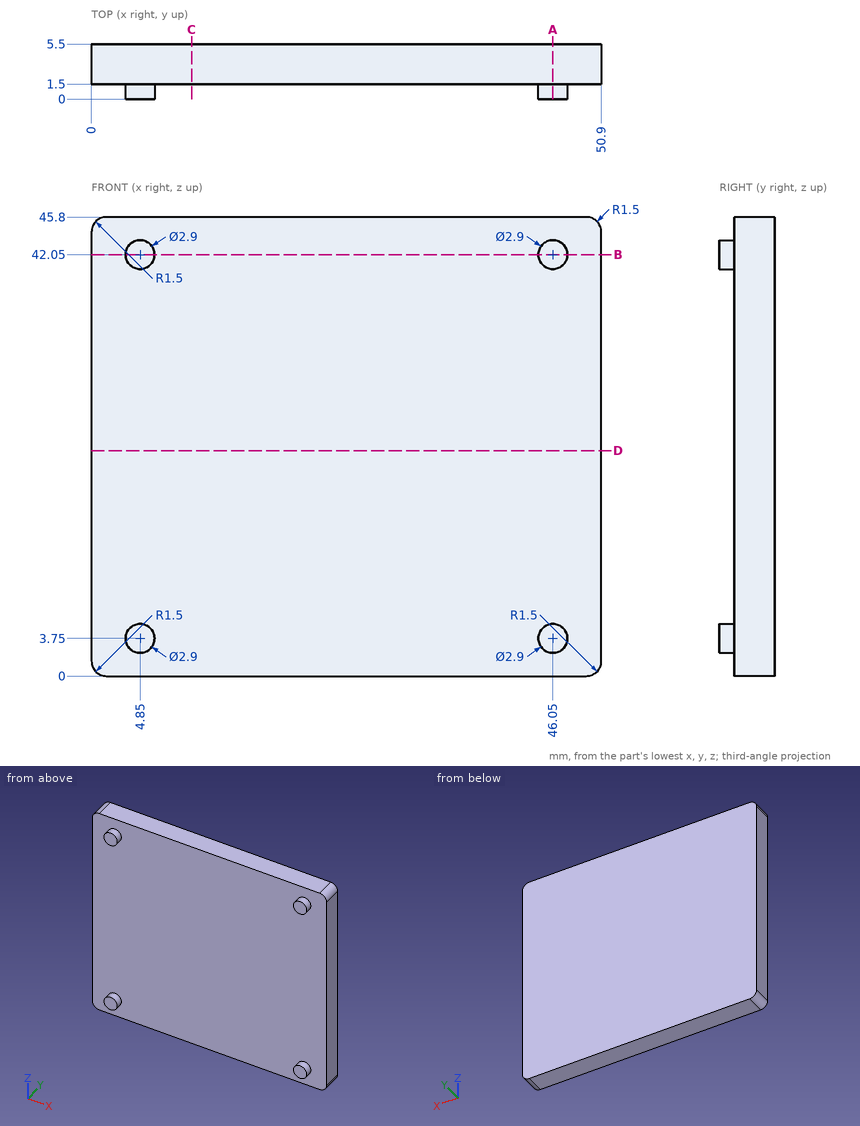
Job drawing, mm, ordinate dimensions from the low corner. One solid piece. Coordinates: 2 decimals unless noted, no trailing zeros. Write each loop counter-clockwise with the first axis right and the second up, starting at its lowest first coordinate (ties: lowest second). Pieces come first, ordered by that corner, then holes.
Item 1: Slice it at D-D (z = 22.5). Write the cut outline in (x, y), and give its area (3 significant figures).
Item 2: Slice it at A-A (x = 46.05). Write the cut outline in (y, z), and give its area (3 significant figures).
Item 3: Probe line 1 (Y direction, x = 9, z = 28). List the from-to ranges inside material, lowest first.
Item 4: Slice it at C-C (x = 10). Write the cut outline in (y, z), and give its area (3 significant figures).
Item 5: Pin check, flat tip, straight feed: pin 1 (13.5 mm diameter, centred on x = 28, z = 25, fed in from -Y). Stop position of the tip, or through.
Item 6: Slice it at B-B (z = 42.05). Write the cut outline in (x, y).
Results found:
1. outline: (0, 1.5) - (50.9, 1.5) - (50.9, 5.5) - (0, 5.5) - close
1. area: 204 mm2
2. outline: (0, 2.3) - (1.5, 2.3) - (1.5, 0) - (5.5, 0) - (5.5, 45.8) - (1.5, 45.8) - (1.5, 43.5) - (0, 43.5) - (0, 40.6) - (1.5, 40.6) - (1.5, 5.2) - (0, 5.2) - close
2. area: 192 mm2
3. line 1: y = 1.5 to 5.5
4. outline: (1.5, 0) - (5.5, 0) - (5.5, 45.8) - (1.5, 45.8) - close
4. area: 183 mm2
5. pin 1: stops at y = 1.5
6. outline: (0, 1.5) - (3.4, 1.5) - (3.4, 0) - (6.3, 0) - (6.3, 1.5) - (44.6, 1.5) - (44.6, 0) - (47.5, 0) - (47.5, 1.5) - (50.9, 1.5) - (50.9, 5.5) - (0, 5.5) - close
